Design review of the part built by this model. Coordinates are the model's own, in mm. Coordinates: 2 decimals unless noted, no trailing zeros. Write each loop counter-clockwise with the first axis right and the second up, starting at its lowest first coordinate (ties: lowest second). Pieces come first, ordered by that corner, then holes.
Q1. Add section D-D, the plane x = 23.8. Give the boundary of the cut face in (y, z), plus the area to 3 significant figures.
Q2. The part is to be moulded in two halves that separate along X. For faces 1 (the face through (-3, 0, 11)), 2 (the face through (0, -6, 3)), 3 (the face through (12.823, 18.837, 1.479)), say which applies: +X half, -X half, draft (parallel to the pull), parting line (faces both ways), or undercut.
Q3. Add section B-B, the plane y = -25. Give the boundary of the cut face in (x, z), plus the area to 3 significant figures.
Q4. Add section C-C, the plane y = 19.5. Give the boundary of the cut face in (x, z), plus the area to 3 significant figures.
Q5. To check wall thickness, follow probe 1 along Z at (x, y) = (-15.5, -15); probe 2 along Y at (x, z) = (23.8, 2.3); probe 3 along X at (y, z) = (-3.5, 2.5). State the ranges of each line that lie inside material, in increasing order.
Q6. Add section A-A, the plane x = 0. Give the boundary of the cut face in (y, z), plus the area to 3 significant figures.
Q7. Clearance check with flat-ended pins moving along their axes: pin 1 Ø5 at (x, y) = (0, 23.8) entering from +Z; pin 2 Ø3.5 at (x, y) = (-20.61, 11.9) entering from -Z; pin 3 Ø5 at (y, z) = (-3, 9.5) entering from -X; pin 4 Ø10 at (y, z) = (-18, 2.5) entering from +X. State where each tip first meets the part, or that it passes through.
from build123d import *

# Parameters (mm, degrees)
SKETCH1_R           = 28.4
SKETCH1_R_2         = 2
BOSS_EXTRUDE1_DEPTH = 3
SKETCH2_R           = 3
BOSS_EXTRUDE2_DEPTH = 16


with BuildPart() as part:
    # Sketch1 → Boss-Extrude1 (new body)
    with BuildSketch(Plane.XY):
        Circle(SKETCH1_R)
        with Locations((23.8, 0)):
            Circle(SKETCH1_R_2, mode=Mode.SUBTRACT)
        with Locations((20.61140461, -11.9)):
            Circle(SKETCH1_R_2, mode=Mode.SUBTRACT)
        with Locations((11.9, -20.61140461)):
            Circle(SKETCH1_R_2, mode=Mode.SUBTRACT)
        with Locations((0, -23.8)):
            Circle(SKETCH1_R_2, mode=Mode.SUBTRACT)
        with Locations((-11.9, -20.61140461)):
            Circle(SKETCH1_R_2, mode=Mode.SUBTRACT)
        with Locations((-20.61140461, -11.9)):
            Circle(SKETCH1_R_2, mode=Mode.SUBTRACT)
        with Locations((-23.8, 0)):
            Circle(SKETCH1_R_2, mode=Mode.SUBTRACT)
        with Locations((-20.61140461, 11.9)):
            Circle(SKETCH1_R_2, mode=Mode.SUBTRACT)
        with Locations((-11.9, 20.61140461)):
            Circle(SKETCH1_R_2, mode=Mode.SUBTRACT)
        with Locations((0, 23.8)):
            Circle(SKETCH1_R_2, mode=Mode.SUBTRACT)
        with Locations((11.9, 20.61140461)):
            Circle(SKETCH1_R_2, mode=Mode.SUBTRACT)
        with Locations((20.61140461, 11.9)):
            Circle(SKETCH1_R_2, mode=Mode.SUBTRACT)
    extrude(amount=BOSS_EXTRUDE1_DEPTH)

    # Sketch2 → Boss-Extrude2 (add)
    with BuildSketch(Plane.XY.offset(3)):
        Circle(SKETCH2_R)
    extrude(amount=BOSS_EXTRUDE2_DEPTH)


solid = part.part
Here are the results:
1. outline: (-15.5, 0) - (-2, 0) - (-2, 3) - (-15.5, 3) - close; (2, 0) - (15.5, 0) - (15.5, 3) - (2, 3) - close
1. area: 81.0 mm2
2. face 1: parting line
2. face 2: draft
2. face 3: undercut
3. outline: (-13.47, 0) - (-1.6, 0) - (-1.6, 3) - (-13.47, 3) - close; (1.6, 0) - (13.47, 0) - (13.47, 3) - (1.6, 3) - close
3. area: 71.2 mm2
4. outline: (-20.65, 0) - (-13.56, 0) - (-13.56, 3) - (-20.65, 3) - close; (-10.24, 0) - (10.24, 0) - (10.24, 3) - (-10.24, 3) - close; (13.56, 0) - (20.65, 0) - (20.65, 3) - (13.56, 3) - close
4. area: 104 mm2
5. probe 1: z = 0 to 3
5. probe 2: y = -15.5 to -2, 2 to 15.5
5. probe 3: x = -28.18 to 28.18
6. outline: (-28.4, 0) - (-25.8, 0) - (-25.8, 3) - (-28.4, 3) - close; (-21.8, 0) - (21.8, 0) - (21.8, 3) - (3, 3) - (3, 19) - (-3, 19) - (-3, 3) - (-21.8, 3) - close; (25.8, 0) - (28.4, 0) - (28.4, 3) - (25.8, 3) - close
6. area: 242 mm2
7. pin 1: stops at z = 3
7. pin 2: passes through
7. pin 3: stops at x = -2.96
7. pin 4: stops at x = 25.25
